For this review, take the finished solid that the model builds, in its own axes (mm). A direction names the side the tool comes from. Round coordinates to 2 decimals unless told otherwise and drop trailing zeros. Write each loop counter-clockwise with the first axis right and the second up, starting at its lowest first coordinate (ties: lowest second). Pieces come first, ordered by that corner, then holes. Notation, with made-up numbers: M 11,-39 L 43,-39 A19 ccw 43,-10 Z; hole C 5,-23.5 d4. An arc over 180 degrees is marked long. Use one line per item in the form item = value. Start each with the question number.
Item 1: Draft analysis for pull direction Y (two halves, no side actions). For faces 1 (the cylindrical face through (34.02, -26.59, -64.86)), 2 (the cylindrical face through (37.08, 46.57, -11.93)), 3 (the flat face through (38, 81, -19.05)), state which applies: released by +Y, released by -Y, zero draft, split by the parting line, or undercut.
Item 2: For P1, Ø2, axis at x = 20.5, z = -14.5, coming from the -Y side; P2, Ø8, axis at x = 15, z = -18, coming from the -Y side; P3, Ø5, axis at y = -22.5, z = -47, coming from the +X side; P4, Ø1.5, axis at x = 26.5, y = 63.5, coming from the +Z side, all flat-tipped, find the tip position at first contact; note any pin that passes through.
Item 3: Add section B-B (y = 59.5). State the section outline as (x, z) points.
Item 4: Add section A-A (z = -37). State the section outline as (x, y) points, and give its area (3 significant figures).
Item 5: For line 1 (Z direction, x = 35.5, y = 53); line 2 (Z direction, x = 40, y = -16) (3 decimals); line 3 (Y direction, x = 4, z = -78), list the stretches that pass through material, from the lowest coordinate up. Write a range as [from, to].
Item 6: Add section D-D (x = 26). Count the separate pieces of the cut face and the enclosed holes in it, and give its area (3 significant figures).
Item 7: Add section C-C (z = -7). State the section outline as (x, y) points.
Item 8: For faces 4 (the cylindrical face through (38.446, 46.322, -20.11)), 5 (the flat face through (23, 72, -2.54)), 6 (the cylindrical face through (20.424, 38.044, -40.524)), list the 3-axis set-ups (+Z, -Z, +X, -X, +Y, -Y) from which the entire face can be reached by the end or side of a thin tool; tool diameter is ignored.
from build123d import *

# Parameters (mm, degrees)
BOSS_EXTRUDE1_DEPTH            = 81.28
SKETCH3_W                      = 76.2
SKETCH3_H                      = 50.292
CUT_EXTRUDE1_DEPTH             = 37.846
SKETCH4_W                      = 40.386
SKETCH4_H                      = 43.18
CUT_EXTRUDE2_DEPTH             = 52.832
FILLET1_R                      = 2.54
FILLET2_R                      = 2.54
FILLET3_R                      = 2.54
FILLET4_R                      = 2.54
SKETCH7_W                      = 16.51
SKETCH7_H                      = 2.54
CUT_EXTRUDE4_REACH             = 54.566
SKETCH8_W                      = 16.51
SKETCH8_H                      = 16.012242806
CUT_EXTRUDE4_DIRECTION_2_DEPTH = 2.54
FILLET5_R                      = 1.27


with BuildPart() as part:
    # Sketch1 → Boss-Extrude1 (new body)
    with BuildSketch(Plane.XY):
        with BuildLine():
            Line((0, 52.959), (0, 58.039))
            ThreePointArc((0, 58.039), (12.7, 70.739), (0, 83.439))
            Line((0, 83.439), (0, 98.679))
            Line((0, 98.679), (40.386, 98.679))
            Line((40.386, 98.679), (40.386, 25.398729968))
            ThreePointArc((40.386, 25.398729968), (40.827682914, 17.344312358), (42.147434783, 9.386487162))
            ThreePointArc((42.147434783, 9.386487162), (33.688432107, -27.011144777), (0, -43.18))
            Line((0, -43.18), (0, -35.179))
            ThreePointArc((0, -35.179), (35.179, 0), (0, 35.179))
            Line((0, 35.179), (0, 52.959))
        make_face()
    extrude(amount=-BOSS_EXTRUDE1_DEPTH)

    # Sketch3 → Cut-Extrude1 (cut)
    with BuildSketch(Plane.ZY):
        with Locations((-40.64, 70.993)):
            Rectangle(SKETCH3_W, SKETCH3_H)
    extrude(amount=-CUT_EXTRUDE1_DEPTH, mode=Mode.SUBTRACT)

    # Sketch4 → Cut-Extrude2 (cut)
    with BuildSketch(Plane(origin=(0, 98.679, 0), x_dir=(1, 0, 0), z_dir=(0, 1, 0))):
        with Locations((20.193, 40.64)):
            Rectangle(SKETCH4_W, SKETCH4_H)
    extrude(amount=-CUT_EXTRUDE2_DEPTH, mode=Mode.SUBTRACT)

    # Fillet1
    fillet1_edges = [part.edges().sort_by_distance(p)[0] for p in [
        (18.923, 45.847, -78.74),
        (18.923, 45.847, -2.54),
        (37.846, 45.847, -10.795),
        (37.846, 45.847, -70.485),
    ]]
    fillet(fillet1_edges, radius=FILLET1_R)

    # Fillet2
    fillet2_edges = [part.edges().sort_by_distance(p)[0] for p in [
        (37.846, 96.139, -70.485),
        (37.846, 96.139, -10.795),
    ]]
    fillet(fillet2_edges, radius=FILLET2_R)

    # Fillet3
    fillet3_edges = [part.edges().sort_by_distance(p)[0] for p in [
        (36.576, 45.847, -19.05),
        (36.576, 45.847, -62.23),
    ]]
    fillet(fillet3_edges, radius=FILLET3_R)

    # Fillet4
    fillet4_edges = [part.edges().sort_by_distance(p)[0] for p in [
        (40.386, 98.679, -71.755),
        (40.386, 98.679, -9.525),
    ]]
    fillet(fillet4_edges, radius=FILLET4_R)

    # Sketch7 → Cut-Revolve2 (revolve, cut)
    with BuildSketch(Plane.ZY):
        with Locations((-40.64, -41.91)):
            Rectangle(SKETCH7_W, SKETCH7_H)
    revolve(axis=Axis((0, 0, -81.28), (0, 0, 1)), mode=Mode.SUBTRACT)

    # Sketch8 → Cut-Extrude4 (cut, up to next)
    with BuildSketch(Plane(origin=(42.147434783, 9.386487162, 0), x_dir=(0, 0, -1), z_dir=(0.976086957, 0.217380435, 0)), mode=Mode.PRIVATE) as cut_extrude4_sk1:
        with Locations((40.64, 8.006121403)):
            Rectangle(SKETCH8_W, SKETCH8_H)
    cut_extrude4_tool1 = extrude(cut_extrude4_sk1.sketch, amount=-CUT_EXTRUDE4_REACH, mode=Mode.PRIVATE) & part.part
    add(cut_extrude4_tool1.solids().sort_by_distance((40.407061, 17.201158, -40.64))[0], mode=Mode.SUBTRACT)

    # Sketch8 → Cut-Extrude4 direction 2 (cut)
    with BuildSketch(Plane(origin=(42.147434783, 9.386487162, 0), x_dir=(0, 0, -1), z_dir=(0.976086957, 0.217380435, 0))):
        with Locations((40.64, 8.006121403)):
            Rectangle(SKETCH8_W, SKETCH8_H)
    extrude(amount=CUT_EXTRUDE4_DIRECTION_2_DEPTH, mode=Mode.SUBTRACT)

    # Fillet5
    fillet5_edges = [part.edges().sort_by_distance(p)[0] for p in [
        (40.64, 0, -48.895),
        (40.64, 0, -32.385),
    ]]
    fillet(fillet5_edges, radius=FILLET5_R)


solid = part.part
Calculated:
q1.face_1 = split by the parting line
q1.face_2 = undercut
q1.face_3 = zero draft
q2.P1 = -38.53
q2.P2 = -41.76
q2.P3 = 37.8
q2.P4 = 0
q3.outline = M 5.91,-81.28 L 40.39,-81.28 L 40.39,-62.23 L 37.85,-62.23 L 37.85,-78.74 L 5.91,-78.74 Z; M 5.91,-2.54 L 37.85,-2.54 L 37.85,-19.05 L 40.39,-19.05 L 40.39,0 L 5.91,0 Z
q4.outline = M 0,-40.64 A40.64 ccw 0,40.64 L 0,35.18 A35.18 cw 0,-35.18 Z; M 0,43.18 A43.18 cw 35.66,24.35 L 40.39,25.4 L 40.39,45.85 L 0,45.85 Z
q4.area = 1,040 mm^2
q5.line_1 = [-81.28, -78.74], [-2.54, 0]
q5.line_2 = [-81.28, -48.895], [-32.385, 0]
q5.line_3 = [-42.99, -34.95], [34.95, 46.59], [96.14, 98.68]
q6.separate_pieces = 2
q6.enclosed_holes = 1
q6.area = 2,930 mm^2
q7.outline = M 0,-43.18 A43.18 ccw 42.15,9.39 A73.66 cw 40.39,25.4 L 40.39,96.14 A2.54 ccw 37.85,98.68 L 0,98.68 L 0,96.14 L 35.31,96.14 A2.54 cw 37.85,93.6 L 37.85,48.39 A2.54 cw 35.31,45.85 L 0,45.85 L 0,35.18 A35.18 cw 0,-35.18 Z
q8.face_4 = +X, -X, +Y
q8.face_5 = -X
q8.face_6 = none
